Build history of the part. All positions in model axes, mm. A direction names the side the tool comes from. Give positions to 0.01 mm unless a question says otherwise; leave off trailing zeros. Write each loop counter-clockwise with the first axis right and the second up, starting at its lowest first coordinate (ties: lowest second). Pieces come first, ordered by that corner, then holes. Notation, with made-up numbers: (54.25, -29) -> (75.25, -29) arc R32 ccw to (75.25, 9) -> close; hole circle Ø3 at (-24, 8). An arc over 180 degrees is marked (long way). Write item = value, one per line. Start each with the question number.
Q1. Drop flat-ended pins along their axis: P1, Ø5.5, axis at y = 9, z = -16, coming from the +X side; P2, Ø5.5, axis at x = -10.5, y = 9.5, coming from the +Z side; P3, Ø3, axis at x = -13, z = -15, coming from the -Y side; P4, Ø5, axis at x = -13.5, z = -7, coming from the -Y side. Give the stop position or say it passes through.
Q2. Saw through at B-B, the plane y = 8.5. List the corners of the cut face in (x, z), then the cut area to 3 significant figures.
Q3. Saw through at D-D, the plane x = -11.75. List the corners of the cut face in (y, z), then the cut area to 3 significant figures.
Q4. Saw through at C-C, the plane z = -21.5. List the corners of the cut face in (x, y), then the cut area to 3 significant figures.
Q5. Mould opens along X. For faces 1 (the face through (-0.81, 2.54, -2.38)), 2 (the face through (-5, 5, -15)), 3 (the face through (-16.881, 8, -7)) say: pulls with the +X half, pulls with the -X half, needs draft (parallel to the pull), parting line crosses it, or undercut.
Q6. Saw through at A-A, the plane x = -2. List the corners of the cut face in (y, z).
Q7. Wall check: line 1 (Z direction, x = -2, y = 3); line 2 (Z direction, x = -14.75, y = 6.5); line 3 (X direction, y = 3.9, z = -2). Give the ranges that are in metal, low to high.
Q8. Tool access for faces 4 (the face through (-10, 5, -15)), 5 (the face through (-12, 8, -5)), 6 (the face through (-13, 5, -23)): list every direction of +Z, -Z, +X, -X, +Y, -Y with a clear straight run to the whole face (end or side of a thin tool).
Autodesk Inventor part; units mm, degrees
ref_plane "YZ Plane" through (0, 0, 0) normal (1, 0, 0) x (0, 1, 0)
ref_plane "XZ Plane" through (0, 0, 0) normal (0, 1, 0) x (-1, 0, 0)
ref_plane "XY Plane" through (0, 0, 0) normal (0, 0, 1) x (1, 0, 0)
sketch "Sketch1" plane through (0, 0, 0) normal (0, 1, 0) x (-1, 0, 0)
  line L0 (0, 0) -> (10, 0)
  line L1 (10, 0) -> (10, -30)
  line L2 (10, -30) -> (0, -30)
  line L3 (0, -30) -> (0, 0)
  dimension "d0" = 30
  dimension "d1" = 10
extrude "Extrusion1" add sketch "Sketch1" along normal blind 5
sketch "Sketch2" plane through (0, 5, 0) normal (0, 1, 0) x (1, 0, 0)
  circle A0 centre (-2, 2) radius 1.25
  circle A1 centre (-2, 25.4965) radius 1.25
  line L0 (0, 0) -> (0, 30)
  line L1 (-10, 0) -> (0, 0)
  dimension "d4" = 2.5
  dimension "d5" = 2.5
  dimension "d6" = 23.4965
  dimension "d7" = 2
  dimension "d8" = 2
extrude "Extrusion2" cut sketch "Sketch2" against normal through all
sketch "Sketch3" plane through (0, 5, 0) normal (0, 1, 0) x (1, 0, 0)
  line L0 (-10, 30) -> (-10, 0)
  line L1 (-10, 5) -> (-10, 25)
  line L2 (-10, 25) -> (-16.8813, 25)
  line L3 (-16.8813, 25) -> (-16.8813, 5)
  line L4 (-16.8813, 5) -> (-10, 5)
  line L5 (-7.2371, 5) -> (-7.2371, 25)
  line L6 (-7.2371, 25) -> (-10, 25)
  line L7 (-10, 5) -> (-7.2371, 5)
  line L8 (-10, 0) -> (0, 0)
  dimension "d11" = 20
  dimension "d22" = 5
extrude "Extrusion3" add sketch "Sketch3" along normal blind 7
sketch "Sketch4" plane through (-10, 5, -25) normal (0, 0, -1) x (-1, 0, 0)
  circle A0 centre (4.3813, 3.5) radius 2
  line L0 (6.8813, 0) -> (6.8813, 7)
  point P0 (-10, -5)
  dimension "d14" = 4
  dimension "d15" = 2.5
extrude "Extrusion4" cut sketch "Sketch4" against normal through all
sketch "Sketch5" plane through (0, 12, 0) normal (0, 1, 0) x (1, 0, 0)
  line L0 (-16.8813, 25) -> (-16.8813, 5)
  line L1 (-10, 30) -> (-10, 0)
  line L2 (-16.8813, 10) -> (-10, 10)
  line L3 (-10, 10) -> (-10, 19.25)
  line L4 (-10, 19.25) -> (-16.8813, 19.25)
  line L5 (-16.8813, 19.25) -> (-16.8813, 10)
  line L6 (-16.8813, 5) -> (-7.2371, 5)
  point P0 (0, 0)
  point P1 (-16.8813, 19.25)
  point P2 (-10, 10)
  dimension "d18" = 9.25
  dimension "d19" = 5
extrude "Extrusion5" cut sketch "Sketch5" against normal through all contours L4 L1 L2 L0
sketch "Sketch6" plane through (0, 12, 0) normal (0, 1, 0) x (1, 0, 0)
  line L0 (-16.8813, 10) -> (-16.8813, 5)
  line L1 (-10, 30) -> (-10, 0)
  line L2 (-16.8813, 9.3856) -> (-10, 9.3856)
  line L3 (-10, 9.3856) -> (-10, 20.0346)
  line L4 (-10, 20.0346) -> (-16.8813, 20.0346)
  line L5 (-16.8813, 20.0346) -> (-16.8813, 9.3856)
  point P0 (0, 0)
extrude "Extrusion6" cut sketch "Sketch6" against normal through all
properties part number "test hålare_3DPrint"
Report:
q1.P1 = -7.24
q1.P2 = -5
q1.P3 = through
q1.P4 = 5
q2.outline = (-16.88, -25) -> (-16.38, -25) -> (-16.38, -20.03) -> (-16.88, -20.03) -> close; (-16.88, -9.39) -> (-16.38, -9.39) -> (-16.38, -5) -> (-16.88, -5) -> close; (-12.38, -25) -> (-7.24, -25) -> (-7.24, -5) -> (-12.38, -5) -> (-12.38, -9.39) -> (-10, -9.39) -> (-10, -20.03) -> (-12.38, -20.03) -> close
q2.area = 82.2 mm2
q3.outline = (5, -25) -> (12, -25) -> (12, -20.03) -> (5, -20.03) -> close; (5, -9.39) -> (12, -9.39) -> (12, -5) -> (5, -5) -> close
q3.area = 65.5 mm2
q4.outline = (-16.88, 5) -> (-10, 5) -> (-10, 0) -> (0, 0) -> (0, 5) -> (-7.24, 5) -> (-7.24, 12) -> (-16.88, 12) -> close; hole circle Ø4 at (-14.38, 8.5)
q4.area = 105 mm2
q5.face_1 = undercut
q5.face_2 = needs draft
q5.face_3 = pulls with the -X half
q6.outline = (0, -30) -> (5, -30) -> (5, -26.75) -> (0, -26.75) -> close; (0, -24.25) -> (5, -24.25) -> (5, -3.25) -> (0, -3.25) -> close; (0, -0.75) -> (5, -0.75) -> (5, 0) -> (0, 0) -> close
q7.line_1 = -30 to -26.75, -24.25 to -3.25, -0.75 to 0
q7.line_2 = -25 to -20.03, -9.39 to -5
q7.line_3 = -10 to -3.25, -0.75 to 0
q8.face_4 = -X, -Y
q8.face_5 = +Z, +X, -X, +Y
q8.face_6 = +Z, -Z, -X, -Y
